from build123d import *

# Parameters (mm, degrees)
F0_W     = 1116.0125
F0_H     = 207.01
F1_DEPTH = 19.05
F2_W     = 6.35
F2_H     = 6.35
F3_DEPTH = 1116.0135
F4_W     = 6.35
F4_H     = 6.35
F5_DEPTH = 1116.0135


with BuildPart() as f1:
    # F0 (on Front) → F1 (new body)
    with BuildSketch(Plane.XZ):
        with Locations((-41.97727, -399.287407)):
            Rectangle(F0_W, F0_H)
    extrude(amount=F1_DEPTH)

    # F2 (on face) → F3 (cut, through all)
    with BuildSketch(Plane.YZ.offset(516.02898)):
        with Locations((-9.525, -298.957407)):
            Rectangle(F2_W, F2_H)
    extrude(amount=-F3_DEPTH, mode=Mode.SUBTRACT)

    # F4 (on face) → F5 (cut, through all)
    with BuildSketch(Plane.YZ.offset(516.02898)):
        with Locations((-15.875, -499.617407)):
            Rectangle(F4_W, F4_H)
        with Locations((-3.175, -499.617407)):
            Rectangle(F4_W, F4_H)
    extrude(amount=-F5_DEPTH, mode=Mode.SUBTRACT)


solid = f1.part
Geometry check sheet. Reference: the model listing, model coordinates, mm. Give positions to 0.01 mm unless a question says otherwise; leave off trailing zeros. Write each loop counter-clockwise with the first axis right and the second up, starting at its lowest first coordinate (ties: lowest second). Pieces come first, ordered by that corner, then holes.
1) Release check for a two-part mould opening along Y. For faces 1 (the face through (-50, 0, -395)), 2 (the face through (-599.984, -9, -401)), 3 (the face through (-50, -19.05, -395)) record: released by +Y, released by -Y, zero draft, split by the parting line, or undercut.
Values follow:
face 1: released by +Y
face 2: zero draft
face 3: released by -Y
2) Go/stop test with flat-tipped pins: pin 1 Ø7 at (x, z) = (-228.5, -500) entering from +Y; pin 2 Ø3 at (x, y) = (-246, -8) entering from +Z; pin 3 Ø5 at (x, z) = (48, -499) entering from -Y. Record where each tip stops, or that it passes through.
Values follow:
pin 1: stops at y = -6.35
pin 2: stops at z = -302.13
pin 3: stops at y = -12.7
3) Cross-section at B-B (y = -9.5). Record the boundary of the cut face in (x, z).
Values follow:
outline: (-599.98, -502.79) - (516.03, -502.79) - (516.03, -302.13) - (-599.98, -302.13) - close
4) Cross-section at A-A (x = 339). Record the boundary of the cut face in (y, z).
Values follow:
outline: (-19.05, -496.44) - (-12.7, -496.44) - (-12.7, -502.79) - (-6.35, -502.79) - (-6.35, -496.44) - (0, -496.44) - (0, -295.78) - (-6.35, -295.78) - (-6.35, -302.13) - (-12.7, -302.13) - (-12.7, -295.78) - (-19.05, -295.78) - close
5) Thickness scan on line 1 (Z direction, x = -189, y = -5.5); line 2 (Z direction, x = -254, y = -12). Record the ranges inside material, lowest first.
Values follow:
line 1: z = -496.44 to -295.78
line 2: z = -502.79 to -302.13
